from build123d import *

# Parameters (mm, degrees)
SKETCH2_W               = 5
SKETCH2_H               = 7.5
BOSS_EXTRUDE1_DEPTH     = 5
CUT_EXTRUDE1_DEPTH      = 7.731456009
CUT_EXTRUDE1_DEPTH_BACK = 5


with BuildPart() as part:
    # Sketch2 → Boss-Extrude1 (new body)
    with BuildSketch(Plane(origin=(0, 0, 0), x_dir=(1, 0, 0), z_dir=(0, 1, 0))):
        Rectangle(SKETCH2_W, SKETCH2_H)
    extrude(amount=BOSS_EXTRUDE1_DEPTH)

    # Sketch3 → Cut-Extrude1 (cut, two sides: drawn at the far end of the back side and taken through both)
    with BuildSketch(Plane.XZ.offset(-CUT_EXTRUDE1_DEPTH_BACK)):
        Polygon((-26.642135624, -1.25), (-2.5, -1.25), (0, -1.25), (0, 2.25), (-2, 2.25), (-2, 1.25), (-2.5, 1.25), (-26.642135624, 1.25), (-74.926406871, 1.25), (-74.926406871, -1.25), align=None)
    extrude(amount=CUT_EXTRUDE1_DEPTH + CUT_EXTRUDE1_DEPTH_BACK, mode=Mode.SUBTRACT)


solid = part.part
Geometry check sheet. Reference: the model listing, model coordinates, mm. A direction names the side the tool comes from. Round coordinates to 2 decimals unless told otherwise and drop trailing zeros. Loops run counter-clockwise (first coordinate to the right, second up) from the corner with the lowest first, then second, coordinate; pieces in that order, holes last. Notation, with made-up numbers: (-1.5, -8.5) - (35.5, -8.5) arc R33 ccw to (35.5, 21.5) - close; hole circle Ø1 at (17, -25). An arc over 180 degrees is marked (long way). One line per question, with ' | ' between items. Start each with the question number.
1. Tool access check on faces 1 (the face through (-1, 3, -1.25)), 2 (the face through (0, 2, -3.75)), 3 (the face through (-1, 3, 2.25)). Record the directions out of +Z, -Z, +X, -X, +Y, -Y that give a thin tool (end or side, any length) a straight path to the whole face; none if there is none.
2. Scan lines: line 1 (Z direction, x = -1.5, y = 2.9); line 2 (X direction, y = 2.05, z = 1.75); line 3 (X direction, y = 0.35, z = -0.75). Record each from-to range of solid material in increasing order. Write a range as [from, to].
3. Cross-section at C-C on y = 2.3. Record the cut outline in (x, z), then the cut area to 4 significant figures.
4. Cross-section at B-B on z = 1.5. Record the cut outline in (x, y), then the cut area to 3 significant figures.
5. Cross-section at A-A on x = -0.5. Record the cut outline in (y, z), then the cut area to 3 significant figures.
6. Cross-section at D-D on z = -1. Record the cut outline in (x, y), then the cut area to 3 significant figures.
7. Draft check along Z on faces 4 (the face through (-2.5, 2, -2)), 5 (the face through (-2, 3, 2)), 6 (the face through (0, 2, 3.75)). Enter one of: released by +Z, released by -Z, zero draft, split by the parting line, or undercut.
Taken from the geometry:
1) face 1: -X, +Y, -Y | face 2: -Z, +X, -X, +Y, -Y | face 3: +Y, -Y
2) line 1: [-3.75, -1.25], [2.25, 3.75] | line 2: [-2.5, -2], [0, 2.5] | line 3: [0, 2.5]
3) outline: (-2.5, -3.75) - (2.5, -3.75) - (2.5, 3.75) - (-2.5, 3.75) - (-2.5, 1.25) - (-2, 1.25) - (-2, 2.25) - (0, 2.25) - (0, -1.25) - (-2.5, -1.25) - close | area: 29.25 mm²
4) outline: (-2.5, 0) - (-2, 0) - (-2, 5) - (-2.5, 5) - close; (0, 0) - (2.5, 0) - (2.5, 5) - (0, 5) - close | area: 15.0 mm²
5) outline: (0, -3.75) - (5, -3.75) - (5, -1.25) - (0, -1.25) - close; (0, 2.25) - (5, 2.25) - (5, 3.75) - (0, 3.75) - close | area: 20.0 mm²
6) outline: (0, 0) - (2.5, 0) - (2.5, 5) - (0, 5) - close | area: 12.5 mm²
7) face 4: zero draft | face 5: undercut | face 6: released by +Z
